Verification items for the finished model (mm, model axes). A direction names the side the tool comes from. Round coordinates to 2 decimals unless told otherwise and drop trailing zeros. Write each loop counter-clockwise with the first axis right and the second up, starting at its lowest first coordinate (ties: lowest second). Pieces come first, ordered by that corner, then holes. Notation, with made-up numbers: M -19,22.25 L 10,22.25 A22 ccw 10,37.25 Z; hole C 75.25,43.5 d6. An arc over 180 degrees is marked long. One line per question, with ' | ' between items. Start each with the question number.
Q1. Tool access check on faces 1 (the face through (-5, -2, 3)), 2 (the face through (-3.145, -3.742, 3.451)), 3 (the face through (4.05, -1, 3)), 4 (the face through (2.8, -2, 3)). Record the directions out of +Z, -Z, +X, -X, +Y, -Y that give a thin tool (end or side, any length) a straight path to the whole face; none if there is none.
Q2. Cross-section at C-C (x = 3.25). Record the boundary of the cut face in (y, z).
Q3. Cross-section at B-B (y = -1.5). Record the boundary of the cut face in (x, z).
Q4. Gauge pin test, flat ends, axial feed: pin 1 (2 mm diameter, centred on y = -4, z = 2, fed in from -X); pin 2 (1.6 mm diameter, centred on x = 4.5, z = 5, fed in from -Y); pin 3 (2 mm diameter, centred on y = -5, z = 5, fed in from +X). Record the tip position at first contact, or that the pin passes through.
Q5. Thickness scan on line 1 along X through (y, z) = (-1.75, 1.5); line 2 along X through (y, z) = (-4.5, 2.5); line 3 along X through (y, z) = (-2.75, 6.75). Record the ranges inside material, lowest first. Write a range as from..to.
Q6. Cross-section at A-A (y = -2.75). Record the boundary of the cut face in (x, z).
Q7. Cross-section at D-D (z = 6). Record the boundary of the cut face in (x, y), then the cut area to 3 significant figures.
from build123d import *

# Parameters (mm, degrees)
F1_DEPTH = 7
F2_SIZE  = 1


with BuildPart() as f1:
    # F0 (on Top) → F1 (new body)
    with BuildSketch(Plane.XY):
        Polygon((-0.9, -7.4), (-0.9, 0), (-2.8, 0), (-2.8, -3.200004), (-2.8, -7.4), align=None)
        Polygon((-2.8, 0), (-0.9, 0), (0.9, 0), (2.8, 0), (4.05, 0), (4.05, -2), (5.55, -2), (5.55, 2), (0, 2), (-5.55, 2), (-5.55, -2), (-4.05, -2), (-4.05, 0), align=None)
        Polygon((2.8, 0), (0.9, 0), (0.9, -7.4), (2.8, -7.4), (2.8, -3.200004), align=None)
        Polygon((-2.8, -7.4), (-2.8, -3.200004), (-3.5, -4.300002), (-3.5, -6.300002), align=None)
        Polygon((2.8, -3.200004), (2.8, -7.4), (3.5, -6.300002), (3.5, -4.300002), align=None)
    extrude(amount=F1_DEPTH)

    # F2
    f2_edges = [f1.edges().sort_by_distance(p)[0] for p in [
        (-5.55, 2, 3.5),
        (5.55, 2, 3.5),
    ]]
    chamfer(f2_edges, length=F2_SIZE)


solid = f1.part
Determined:
1) face 1: +Z, -Z, -X, -Y | face 2: +Z, -Z, -X | face 3: +Z, -Z, -Y | face 4: +Z, -Z
2) outline: M -6.69,0 L -3.91,0 L -3.91,7 L -6.69,7 Z; M 0,0 L 2,0 L 2,7 L 0,7 Z
3) outline: M -5.55,0 L -4.05,0 L -4.05,7 L -5.55,7 Z; M -2.8,0 L -0.9,0 L -0.9,7 L -2.8,7 Z; M 0.9,0 L 2.8,0 L 2.8,7 L 0.9,7 Z; M 4.05,0 L 5.55,0 L 5.55,7 L 4.05,7 Z
4) pin 1: stops at x = -3.5 | pin 2: stops at y = -2 | pin 3: stops at x = 3.5
5) line 1: x = -5.55..-4.05, -2.8..-0.9, 0.9..2.8, 4.05..5.55 | line 2: x = -3.5..-0.9, 0.9..3.5 | line 3: x = -2.8..-0.9, 0.9..2.8
6) outline: M -2.8,0 L -0.9,0 L -0.9,7 L -2.8,7 Z; M 0.9,0 L 2.8,0 L 2.8,7 L 0.9,7 Z
7) outline: M -5.55,-2 L -4.05,-2 L -4.05,0 L -2.8,0 L -2.8,-3.2 L -3.5,-4.3 L -3.5,-6.3 L -2.8,-7.4 L -0.9,-7.4 L -0.9,0 L 0.9,0 L 0.9,-7.4 L 2.8,-7.4 L 3.5,-6.3 L 3.5,-4.3 L 2.8,-3.2 L 2.8,0 L 4.05,0 L 4.05,-2 L 5.55,-2 L 5.55,1 L 4.55,2 L -4.55,2 L -5.55,1 Z | area: 59.7 mm²
